```python
from build123d import *

# Parameters (mm, degrees)
ESQUISSE1_R        = 1.5
BOSS_EXTRU_1_DEPTH = 5
BOSS_EXTRU_2_DEPTH = 5


with BuildPart() as part:
    # Esquisse1 → Boss.-Extru.1 (new body)
    with BuildSketch(Plane.XY):
        Polygon((0, 0), (37, 0), (37, 18), (12, 18), (12, 55), (0, 55), align=None)
        with Locations((6, 32)):
            Circle(ESQUISSE1_R, mode=Mode.SUBTRACT)
        with Locations((31, 12)):
            Circle(ESQUISSE1_R, mode=Mode.SUBTRACT)
    extrude(amount=BOSS_EXTRU_1_DEPTH)

    # Esquisse2 → Boss.-Extru.2 (add)
    with BuildSketch(Plane.XY.offset(5)):
        Polygon((37, 0), (42, 0), (42, -5), (49.5, -5), (49.5, 0), (64.5, 0), (64.5, -5), (72, -5), (72, 0), (79.5, 0), (79.5, 5), (67, 5), (67, 9), (42, 9), (42, 18), (37, 18), align=None)
        Polygon((0, 0), (-17, 0), (-17, 5), (-39, 5), (-39, 15), (-17, 15), (-17, 40), (-39, 40), (-39, 50), (-17, 50), (-17, 55), (0, 55), align=None)
    extrude(amount=-BOSS_EXTRU_2_DEPTH)


solid = part.part
```
CAD build for the part. Positions are in the model's coordinates, mm. A direction names the side the tool comes from. Round coordinates to 2 decimals unless told otherwise and drop trailing zeros. Write each loop counter-clockwise with the first axis right and the second up, starting at its lowest first coordinate (ties: lowest second). Pieces come first, ordered by that corner, then holes. Notation, with made-up numbers: (13.25, 76) - (32.25, 76) arc R21 ccw to (32.25, 91) - close; hole circle Ø3 at (-6, 19.25). An arc over 180 degrees is marked (long way). Write item = value, one per line. Start each with the question number.
Q1. Band-saw the part on D-D (x = 56). Give the cut face in (y, z).
Q2. Probe L1, parallel to X at y = -2, z = 4.25; L2, parallel to Y at x = -18, z = 0.2; L3, parallel to Y at x = 31, z = 1.45. List the from-to ranges inside material, lowest first. Write a range as from..to.
Q3. Band-saw the part on C-C (y = 12). Give the cut face in (x, z), then the cut area to 3 significant figures.
Q4. Band-saw the part on A-A (z = 2.2). Give the cut face in (x, y), then the cut area to 3 significant figures.
Q5. Band-saw the part on B-B (x = 31). Give the cut face in (y, z).
Q6. Mould opens along Y. For faces 5 (the flat face through (-28, 40, 3)), 6 (the flat face through (49.5, -3, 3)), 7 (the flat face through (57, 0, 3)), 8 (the flat face through (73, 5, 3)) say: pulls with the +Y half, pulls with the -Y half, needs draft (parallel to the pull), parting line crosses it, or undercut.
Q7. Which spindle directions (+Z, -Z, +X, -X, +Y, -Y) get a long thin tool onto all of the face, cutting with end or side? Do faces 1 (the flat face through (-28, 50, 3)), 2 (the flat face through (64.5, -2, 3)), 3 (the flat face through (72, -3, 3)), 4 (the flat face through (12, 36, 2)). Say none if no direction does.
Q8. Drop flat-ended pins along their axis: pin 1 (1.5 mm diameter, centred on x = 74, z = 3.5, fed in from +Y); pin 2 (1.5 mm diameter, centred on x = 54, z = 3.5, fed in from +Y); pin 3 (2.5 mm diameter, centred on x = -26.5, z = 2.5, fed in from +Y). Give the stop position or say it passes through.
Answers below:
q1.outline = (0, 0) - (9, 0) - (9, 5) - (0, 5) - close
q2.L1 = 42..49.5, 64.5..72
q2.L2 = 5..15, 40..50
q2.L3 = 0..10.5, 13.5..18
q3.outline = (-39, 0) - (29.5, 0) - (29.5, 5) - (-39, 5) - close; (32.5, 0) - (42, 0) - (42, 5) - (32.5, 5) - close
q3.area = 390 mm2
q4.outline = (-39, 5) - (-17, 5) - (-17, 0) - (42, 0) - (42, -5) - (49.5, -5) - (49.5, 0) - (64.5, 0) - (64.5, -5) - (72, -5) - (72, 0) - (79.5, 0) - (79.5, 5) - (67, 5) - (67, 9) - (42, 9) - (42, 18) - (12, 18) - (12, 55) - (-17, 55) - (-17, 50) - (-39, 50) - (-39, 40) - (-17, 40) - (-17, 15) - (-39, 15) - close; hole circle Ø3 at (6, 32); hole circle Ø3 at (31, 12)
q4.area = 2,920 mm2
q5.outline = (0, 0) - (10.5, 0) - (10.5, 5) - (0, 5) - close; (13.5, 0) - (18, 0) - (18, 5) - (13.5, 5) - close
q6.face_5 = undercut
q6.face_6 = needs draft
q6.face_7 = pulls with the -Y half
q6.face_8 = pulls with the +Y half
q7.face_1 = +Z, -Z, -X, +Y
q7.face_2 = +Z, -Z, -Y
q7.face_3 = +Z, -Z, +X, -Y
q7.face_4 = +Z, -Z, +X, +Y
q8.pin_1 = 5
q8.pin_2 = 9
q8.pin_3 = 50
